```python
from build123d import *

# Parameters (mm, degrees)
F0_R       = 9.525
F0_R_2     = 7.62
F1_DEPTH   = 10.16
F2_SIZE2   = 1.333885
F2_SIZE    = 1.90499
F2_2_SIZE2 = 1.333885
F2_2_SIZE  = 1.90499


# Not quite as in the source:
# - a fillet or chamfer is up to 0.001 mm smaller than in the source, because OpenCascade refuses the exact size


with BuildPart() as f1:
    # F0 (on Front) → F1 (new body)
    with BuildSketch(Plane.XZ):
        Circle(F0_R)
        Circle(F0_R_2, mode=Mode.SUBTRACT)
    extrude(amount=F1_DEPTH)

    # F2 (size 1.905 and 1.3338953603 in the source; OpenCascade refuses exactly that, so slightly less here)
    f2_edges = [f1.edges().sort_by_distance(p)[0] for p in [
        (-9.525, -10.16, 0),
    ]]
    f2_side = f1.faces().sort_by_distance((-9.255592, -10.16, 0))[0]
    chamfer(f2_edges, length=F2_SIZE, length2=F2_SIZE2, reference=f2_side)

    # F2#2 (size 1.905 and 1.3338953603 in the source; OpenCascade refuses exactly that, so slightly less here)
    f2_2_edges = [f1.edges().sort_by_distance(p)[0] for p in [
        (-9.525, 0, 0),
    ]]
    f2_2_side = f1.faces().sort_by_distance((-9.255592, 0, 0))[0]
    chamfer(f2_2_edges, length=F2_2_SIZE, length2=F2_2_SIZE2, reference=f2_2_side)


solid = f1.part
```
Can you work these out from the model? Positions are in its coordinate system, mm. Give positions to 0.01 mm unless a question says otherwise; leave off trailing zeros. Loops run counter-clockwise (first coordinate to the right, second up) from the corner with the lowest first, then second, coordinate; pieces in that order, holes last. Notation, with made-up numbers: M -13,41.5 L 15,41.5 A31 ccw 15,70.5 Z; hole C 5,75.5 d2. An arc over 180 degrees is marked long. One line per question, with ' | ' between items. Start each with the question number.
Q1. If we section it at C-C (y = -6): Please give me the cut outline in (x, z) (3 decimals).
Q2. For pin 1 Ø1 at (y, z) = (-6.5, -7.5) entering from +X; pin 2 Ø2 at (x, y) = (-2, -4.5) entering from +Z; pin 3 Ø1.5 at (y, z) = (-8.5, -1.5) entering from +X, each with a flat end and sliding along its axis, tell me the tip position at first contact or that it passes through.
Q3. If we mould it in two halves opening along X, with no side actions, what happens to faces 1 (the cylindrical face through (-1.65, -5.01, -7.44)), 2 (the cylindrical face through (-7.559, -5.028, -5.796))? For each: +X half, -X half, draft (parallel to the pull), parting line (faces both ways), or undercut.
Q4. If I drill on line 1 (Z direction, x = 0, y = -4.75) (3 decimals); line 2 (X direction, y = -4.75, z = -0.25); line 3 (X direction, y = -1.5, z = 5.5), over which ranges is the centre line in solid material (lowest first)? Write a range as from..to.
Computed:
1) outline: C 0,0 d19.05; hole C 0,0 d15.24
2) pin 1: stops at x = 6.46 | pin 2: stops at z = 9.47 | pin 3: stops at x = 9.5
3) face 1: undercut | face 2: parting line
4) line 1: z = -9.525..-7.62, 7.62..9.525 | line 2: x = -9.52..-7.62, 7.62..9.52 | line 3: x = -7.78..-5.27, 5.27..7.78
